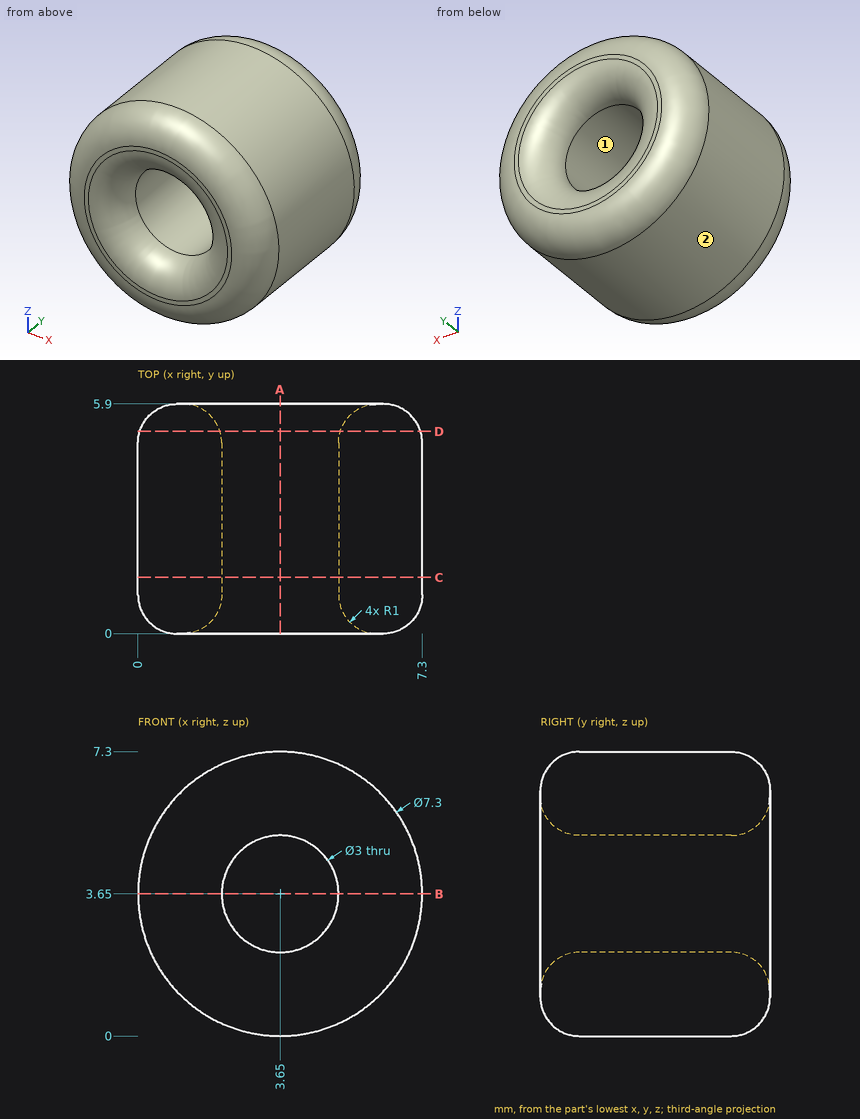
Verification items for this drawing (mm, ordinates from the low corner). Coordinates: 2 decimals unless noted, no trailing zeros. Write each loop counter-clockwise with the first axis right and the second up, starting at its lowest first coordinate (ties: lowest second). Pieces come first, ordered by that corner, then holes. Notation, with made-up numbers: M 81,76.25 L 119,76.25 A26 cw 119,93.25 Z; hole C -12.5,13 d10. An arc over 180 degrees is marked long. Answer as a JSON object with one key per item and string values. Group by question number.
(1) Cross-section at D-D, the plane y = 5.2. Record the cut outline in (x, z), and give its area (3 significant figures).
(2) Gauge pin test, flat ends, axial feed: pin 1 (1.5 mm diameter, centred on y = 2, z = 1, fed in from +X); pin 2 (1.5 mm diameter, centred on x = 1, z = 1, fed in from -Y); pin 3 (2 mm diameter, centred on y = 3.5, z = 6, fed in from +X). Record the tip position at first contact, or that the pin passes through.
(3) Release check for a two-part mould opening along X. For the marked faces 1 and 2 record: +X half, -X half, draft (parallel to the pull), parting line (faces both ways), or undercut.
(4) Material ranges on line 1 (X direction, y = 2.5, z = 3.65); line 2 (Z direction, x = 4.5, y = 3.35); line 3 (Z direction, x = 2.75, y = 3.2), recorded low to high.
(5) Cross-section at B-B, the plane z = 3.65. Record the cut outline in (x, y).
(6) Cross-section at A-A, the plane x = 3.65. Record the cut outline in (y, z), and give its area (3 significant figures).
(7) Cross-section at C-C, the plane y = 1.45. Record the cut outline in (x, z).
Reply:
{
 "1": {"outline": "C 3.65,3.65 d7.21; hole C 3.65,3.65 d3.09", "area": "33.3 mm²"},
 "2": {"pin 1": "x = 6.77", "pin 2": "y = 0.06", "pin 3": "x = 7.04"},
 "3": {"face 1": "undercut", "face 2": "parting line"},
 "4": {"line 1": "0 to 2.15, 5.15 to 7.3", "line 2": "0.1 to 2.41, 4.89 to 7.2", "line 3": "0.11 to 2.45, 4.85 to 7.19"},
 "5": {"outline": "M 0,1 A1 ccw 1,0 L 1.15,0 A1 ccw 2.15,1 L 2.15,4.9 A1 ccw 1.15,5.9 L 1,5.9 A1 ccw 0,4.9 Z; M 5.15,1 A1 ccw 6.15,0 L 6.3,0 A1 ccw 7.3,1 L 7.3,4.9 A1 ccw 6.3,5.9 L 6.15,5.9 A1 ccw 5.15,4.9 Z"},
 "6": {"outline": "M 0,1 A1 ccw 1,0 L 4.9,0 A1 ccw 5.9,1 L 5.9,1.15 A1 ccw 4.9,2.15 L 1,2.15 A1 ccw 0,1.15 Z; M 0,6.15 A1 ccw 1,5.15 L 4.9,5.15 A1 ccw 5.9,6.15 L 5.9,6.3 A1 ccw 4.9,7.3 L 1,7.3 A1 ccw 0,6.3 Z", "area": "23.7 mm²"},
 "7": {"outline": "C 3.65,3.65 d7.3; hole C 3.65,3.65 d3"}
}
